Work out the finished part from the listing and answer in its coordinate system (mm). A direction names the side the tool comes from. Give positions to 0.01 mm unless a question says otherwise; leave off trailing zeros. Write each loop counter-clockwise with the first axis right and the second up, starting at its lowest first coordinate (ties: lowest second). Pieces come first, ordered by that corner, then holes. Notation, with made-up numbers: (49, 77) - (59, 77) arc R19 cw to (59, 82) - close; hole circle Ø1 at (78.25, 32). An arc over 180 degrees is marked (long way). Write item = value, one per line.
from build123d import *

# Parameters (mm, degrees)
SKETCH_1_W         = 20
SKETCH_1_H         = 20
SKETCH_1_W_2       = 16
SKETCH_1_H_2       = 16
EXTRUDE_1_DEPTH    = 550
SKETCH2_R          = 2.5
CUT_EXTRUDE2_DEPTH = 20
SKETCH3_R          = 2
CUT_EXTRUDE3_DEPTH = 20
SKETCH4_R          = 2.5
CUT_EXTRUDE4_DEPTH = 20
SKETCH6_R          = 1.5
CUT_EXTRUDE6_DEPTH = 20
LPATTERN1_COUNT    = 4
LPATTERN1_PITCH    = 120


with BuildPart() as part:
    # 草图1 → 凸台-拉伸1 (new body)
    with BuildSketch(Plane.XY):
        Rectangle(SKETCH_1_W, SKETCH_1_H)
        Rectangle(SKETCH_1_W_2, SKETCH_1_H_2, mode=Mode.SUBTRACT)
    extrude(amount=EXTRUDE_1_DEPTH)

    # Sketch2 → Cut-Extrude2 (cut)
    with BuildSketch(Plane.XZ.offset(10)):
        with Locations(Location((0, 10, 0), (0, 0, 270))):
            Circle(SKETCH2_R)
        with Locations(Location((0, 25, 0), (0, 0, 270))):
            Circle(SKETCH2_R)
    extrude(amount=-CUT_EXTRUDE2_DEPTH, mode=Mode.SUBTRACT)

    # Sketch3 → Cut-Extrude3 (cut)
    with BuildSketch(Plane.ZY.offset(10)):
        with Locations((17.5, 0)):
            Circle(SKETCH3_R)
        with Locations((32.5, 0)):
            Circle(SKETCH3_R)
    extrude(amount=-CUT_EXTRUDE3_DEPTH, mode=Mode.SUBTRACT)

    # Sketch4 → Cut-Extrude4 (cut)
    with BuildSketch(Plane(origin=(10, 0, 0), x_dir=(0, 0, -1), z_dir=(1, 0, 0))):
        with Locations((-540, 0)):
            Circle(SKETCH4_R)
        with Locations((-520, 0)):
            Circle(SKETCH4_R)
        with Locations((-500, 0)):
            Circle(SKETCH4_R)
    extrude(amount=-CUT_EXTRUDE4_DEPTH, mode=Mode.SUBTRACT)

    # Sketch6 → Cut-Extrude6 (cut)
    with BuildSketch(Plane.XZ.offset(10)):
        with Locations(Location((0, 67.5, 0), (0, 0, 270))):
            Circle(SKETCH6_R)
        with Locations(Location((0, 87.5, 0), (0, 0, 270))):
            Circle(SKETCH6_R)
    cut_extrude6 = extrude(amount=-CUT_EXTRUDE6_DEPTH, mode=Mode.SUBTRACT)

    # LPattern1: Cut-Extrude6 ×4
    with Locations(*[(0, 0, i * LPATTERN1_PITCH) for i in range(1, LPATTERN1_COUNT)]):
        add(cut_extrude6, mode=Mode.SUBTRACT)


solid = part.part
1. Find section A-A, the plane z = 337. Give the vertices of the cut face in (x, y).
Solution:
outline = (-10, -10) - (10, -10) - (10, 10) - (-10, 10) - close; hole (-8, -8) - (8, -8) - (8, 8) - (-8, 8) - close
2. Straight lines are drawn through the part: line 1 (X direction, y = -2, z = 167.5); line 2 (X direction, y = -9.3, z = 307.5). For each, find the intervals that lie inside material, in ascending order.
Solution:
line_1 = -10 to -8, 8 to 10
line_2 = -10 to -1.5, 1.5 to 10
3. A tool of negligible diameter and unlimited length cuts with its end or side. For faces 1 (the flat face through (-9, 0, 0)), 2 (the flat face through (0, -8, 271)), from which of +Z, -Z, +X, -X, +Y, -Y can it reach the whole face along a straight path? Write none if from no direction.
Solution:
face_1 = -Z, +X, -X, +Y, -Y
face_2 = +Z, -Z
4. For a pull along Y with two mould halves and no side action, classify faces 3 (the flat face through (8, 0, 271)), 4 (the flat face through (0, -10, 271)), 5 (the flat face through (-9, 0, 550)) as pulls with the +Y half, pulls with the -Y half, needs draft (parallel to the pull), parting line crosses it, or undercut.
Solution:
face_3 = undercut
face_4 = pulls with the -Y half
face_5 = needs draft
